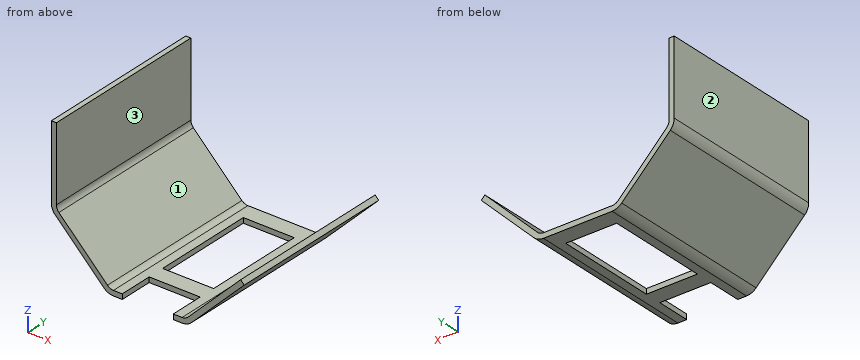
Autodesk Inventor part; units mm, degrees
ref_plane "YZ Plane" through (0, 0, 0) normal (1, 0, 0) x (0, 1, 0)
ref_plane "XZ Plane" through (0, 0, 0) normal (0, 1, 0) x (-1, 0, 0)
ref_plane "XY Plane" through (0, 0, 0) normal (0, 0, 1) x (1, 0, 0)
sketch "Sketch1" plane through (0, 0, 0) normal (0, 0, 1) x (1, 0, 0)
  line L0 (-23.5, -50) -> (23.5, -50)
  line L1 (23.5, -50) -> (23.5, 50)
  line L2 (23.5, 50) -> (-23.5, 50)
  line L3 (-23.5, 50) -> (-23.5, -50)
  line L4 (-23.5, -50) -> (23.5, 50) construction
  line L5 (23.5, -50) -> (-23.5, 50) construction
  point P0 (0, 0)
  dimension "d154" = 47
  dimension "d155" = 100
extrude "Plate3" add sketch "Sketch1" along normal blind 3
sketch "Sketch7" plane through (21.3787, 50, 2.1213) normal (0.7071068, 0, -0.7071068) x (0, 1, 0)
  line L0 (-100, 0) -> (0, 0)
  line L1 (0, 0) -> (0, 47)
  line L2 (0, 47) -> (-100, 47)
  line L3 (-100, 47) -> (-100, 0)
edge flange "Flange3" height 47 angle 45 thickness 3 bend radius 5 thickness toward (0.7071068, 0, -0.7071068) relief round relief width 3 relief depth 1.5 corner gap 5 corner form 0 edges at (23.5, 0, 3) (-23.5, 0, 3) wall of the first edge with corners at (21.3787, -50, 2.1213) (21.3787, 50, 2.1213) (54.6127, 50, 35.3553) (54.6127, -50, 35.3553)
bend "Bend3"
corner "Corner3"
sketch "Sketch8" plane through (0, 0, 3) normal (0, 0, 1) x (1, 0, 0)
  line L0 (15, 40) -> (-15, 40)
  line L1 (-15, 40) -> (-15, -20)
  line L2 (-15, -20) -> (15, -20)
  line L3 (15, -20) -> (15, 40)
  line L4 (15, 40) -> (-15, -20) construction
  line L5 (-15, 40) -> (15, -20) construction
  line L6 (-23.5, 50) -> (20.1863, 50)
  line L7 (-20.1863, -50) -> (20.1863, -50)
  line L8 (15, -50) -> (-15, -50)
  line L9 (-15, -50) -> (-15, -30)
  line L10 (-15, -30) -> (15, -30)
  line L11 (15, -30) -> (15, -50)
  point P0 (0, 0)
  point P1 (0, 10)
  point P2 (-15, -50)
  dimension "d166" = 30
  dimension "d168" = 10
  dimension "d182" = 10
  dimension "d183" = 20
extrude "Cut1" cut sketch "Sketch8" against normal blind 3
sketch "Sketch9" plane through (-53.734, -50, 33.234) normal (-1, 0, 0) x (0, -1, 0)
  line L0 (-100, 0) -> (0, 0)
  line L1 (0, 0) -> (0, 47)
  line L2 (0, 47) -> (-100, 47)
  line L3 (-100, 47) -> (-100, 0)
edge flange "Flange4" height 47 angle 45 thickness 3 bend radius 5 thickness toward (-1, 0, 0) relief round relief width 3 relief depth 1.5 edges at (-54.6127, 0, 35.3553) wall of the first edge with corners at (-53.734, 50, 33.234) (-53.734, -50, 33.234) (-53.734, -50, 80.234) (-53.734, 50, 80.234)
bend "Bend4"
corner "Corner4"
properties part number "DSB-101 Axis" material "Stainless Steel"
Input: part model. Units: mm. Frame: model coordinates. Face numbers are marked on the shaded views. Give positions to 0.01 mm unless a question says otherwise; leave off trailing zeros. Write each loop counter-clockwise with the first axis right and the second up, starting at its lowest first coordinate (ties: lowest second). Pieces come first, ordered by that corner, then holes. Notation, with made-up numbers: (55, -15.75) -> (87, -15.75) arc R12 ccw to (87, -11.75) -> close; hole circle Ø3 at (39.5, -11.5). An arc over 180 degrees is marked (long way). Use one line per item in the form item = value. Start each with the question number.
1) Section query C-C on z = 29. Return the cut outline in (x, y), then the cut area to 3 significant figures.
2) Section query D-D on z = 62. Return the cut outline in (x, y).
3) Draft query along X for the marked faces 1, 2 and 3. Return one class per face: pulls with the +X half, pulls with the -X half, needs draft (parallel to the pull), parting line crosses it, or undercut.
4) Section query A-A on x = 13. Return the cut outline in (y, z), then the cut area to 3 significant figures.
5) Section query B-B on y = -18.5. Return the cut outline in (x, z), then the cut area to 3 significant figures.
6) Ray query, probe 1 along X at (y, z) = (-13, 34); probe 2 along X at (y, z) = (-41, 41.5); probe 3 along X at (y, z) = (13, 8). Return the intervals inside material, ascending. Write a range as from..to.
7) Pin query (flat end, axial travel): pin 1 (1.5 mm diameter, centred on x = -2, z = 1, fed in from -Y); pin 2 (2.5 mm diameter, centred on y = 6.5, z = 2, fed in from +X); pin 3 (2 mm diameter, centred on y = -19.5, z = 34, fed in from -X); pin 4 (2 mm diameter, centred on x = -21, y = -24.5, fed in from -Z). Return the tip coordinate at first contact, or that it passes through.
Outcome:
q1.outline = (-52.5, -50) -> (-48.26, -50) -> (-48.26, 50) -> (-52.5, 50) -> close; (48.26, -50) -> (52.5, -50) -> (52.5, 50) -> (48.26, 50) -> close
q1.area = 849 mm^2
q2.outline = (-56.73, -50) -> (-53.73, -50) -> (-53.73, 50) -> (-56.73, 50) -> close
q3.face_1 = undercut
q3.face_2 = pulls with the -X half
q3.face_3 = pulls with the +X half
q4.outline = (-30, 0) -> (-20, 0) -> (-20, 3) -> (-30, 3) -> close; (40, 0) -> (50, 0) -> (50, 3) -> (40, 3) -> close
q4.area = 60.0 mm^2
q5.outline = (-56.73, 36.55) arc R8 ccw to (-54.39, 30.89) -> (-25.84, 2.34) arc R8 ccw to (-20.19, 0) -> (-15, 0) -> (-15, 3) -> (-20.19, 3) arc R5 cw to (-23.72, 4.46) -> (-52.27, 33.01) arc R5 cw to (-53.73, 36.55) -> (-53.73, 80.23) -> (-56.73, 80.23) -> close; (15, 0) -> (20.19, 0) arc R8 ccw to (25.84, 2.34) -> (56.73, 33.23) -> (54.61, 35.36) -> (23.72, 4.46) arc R5 cw to (20.19, 3) -> (15, 3) -> close
q5.area = 460 mm^2
q6.probe_1 = -56.32..-53.04, 53.26..55.97
q6.probe_2 = -56.73..-53.73
q6.probe_3 = -31.5..-27.26, 27.26..31.5
q7.pin_1 = -30
q7.pin_2 = 26.75
q7.pin_3 = -56.58
q7.pin_4 = 0
